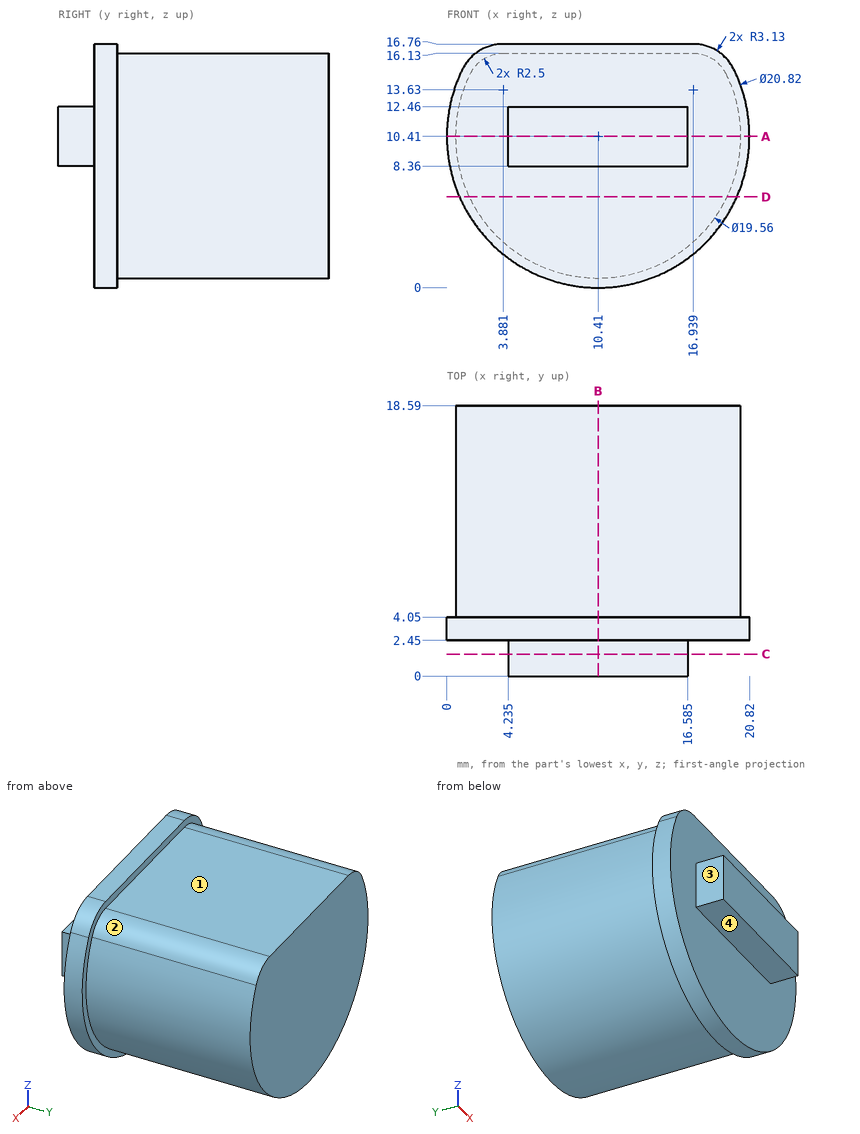
The drawing under review shows one solid part. Ordinate dimensions are in mm from its lowest x, y, z. A direction names the side the tool comes from. Coordinates: 2 decimals unless noted, no trailing zeros. Order: outer loops, then holes, each group sorted by start corner. A loop starts at its lowest first (then second) coordinate and runs counter-clockwise, first axis right, second up. Notation, with made-up numbers: (76.25, 40) -> (124.25, 40) arc R27 cw to (124.25, 68) -> close; hole circle Ø2 at (45.25, 5.25). An arc over 180 degrees is marked (long way). Answer in a Markdown table with one row per item. Add a question column.
Item 1: We need section A-A on z = 10.41. Write out the cut boundary in (x, y) (3 decimals).
Item 2: To check wall thickness, follow probe 1 along Y at (x, z) = (15.5, 13); probe 2 along X at (y, z) = (2, 8.5) (3 decimals); probe 3 along X at (y, z) = (5.25, 5.5). State the ranges of each line that lie inside material, in increasing order.
Item 3: We need section D-D on z = 6.25. Write out the cut boundary in (x, y).
Item 4: Machinability: for the marked faces 1, 2, 3 and 4, which of the approach directions +Z, -Z, +X, -X, +Y, -Y give a long, thin tool a straight path to every point of the face, cutting with its end or side? Answer none if there is none.
Item 5: We need section B-B on x = 10.41. Write out the cut boundary in (y, z).
Item 6: Clearance check with flat-ended pins moving along their axes: pin 1 (3 mm diameter, centred on y = 14, z = 13.5, fed in from +X); pin 2 (2 mm diameter, centred on y = 0.5, z = 11, fed in from +X) (3 decimals); pin 3 (2 mm diameter, centred on x = 9, y = 8, fed in from +Z). State where each tip first meets the part, or that it passes through.
Item 7: We need section C-C on y = 1.5. Write out the cut boundary in (x, z) (3 decimals).
Final values:
| question | item | result |
|---|---|---|
| 1 | outline | (0, 2.45) -> (4.235, 2.45) -> (4.235, 0) -> (16.585, 0) -> (16.585, 2.45) -> (20.82, 2.45) -> (20.82, 4.05) -> (20.19, 4.05) -> (20.19, 18.59) -> (0.63, 18.59) -> (0.63, 4.05) -> (0, 4.05) -> close |
| 2 | probe 1 | y = 2.45 to 18.59 |
| 2 | probe 2 | x = 4.235 to 16.585 |
| 2 | probe 3 | x = 1.95 to 18.87 |
| 3 | outline | (0.87, 2.45) -> (19.95, 2.45) -> (19.95, 4.05) -> (19.26, 4.05) -> (19.26, 18.59) -> (1.56, 18.59) -> (1.56, 4.05) -> (0.87, 4.05) -> close |
| 4 | face 1 | +Z, +X, -X, +Y |
| 4 | face 2 | +Z, +X, +Y |
| 4 | face 3 | +Z, -Z, -X, -Y |
| 4 | face 4 | -Z, +X, -X, -Y |
| 5 | outline | (0, 8.36) -> (2.45, 8.36) -> (2.45, 0) -> (4.05, 0) -> (4.05, 0.63) -> (18.59, 0.63) -> (18.59, 16.13) -> (4.05, 16.13) -> (4.05, 16.76) -> (2.45, 16.76) -> (2.45, 12.46) -> (0, 12.46) -> close |
| 6 | pin 1 | stops at x = 20.06 |
| 6 | pin 2 | stops at x = 16.585 |
| 6 | pin 3 | stops at z = 16.13 |
| 7 | outline | (4.235, 8.36) -> (16.585, 8.36) -> (16.585, 12.46) -> (4.235, 12.46) -> close |
